Can you work these out from the model? Positions are in its coordinate system, mm. A direction names the side the tool comes from. Coordinates: 2 decimals unless noted, no trailing zeros. Order: outer loops, then holes, each group sorted by start corner. A loop starts at its lowest first (then second) coordinate and runs counter-clockwise, first axis right, second up. Notation, with made-up numbers: (45.25, 75) -> (70.25, 75) arc R16 ccw to (70.25, 87) -> close; hole circle Ø1 at (43.5, 72.5). An arc over 180 degrees is marked (long way). Answer as a JSON object with one key per item and string values. Group by question number.
(1) I want a section at A-A, the plane y = -3.5. List the corners of the cut face in (x, z) for me.
(2) I want a section at D-D, the plane y = 2.75. List the corners of the cut face in (x, z) for me.
(3) I want a section at B-B, the plane x = 19. List the corners of the cut face in (y, z) for me.
(4) If we mould it in two halves opening along Z, with no side actions, what happens to faces 1 (the flat face through (5, -12.83, 8)), 2 (the flat face through (5, -7, 0)), 3 (the cylindrical face through (21.432, -12.826, 7.152)), 4 (the cylindrical face through (5.09, -6.73, 1.27))? For each: pulls with the +Z half, pulls with the -Z half, needs draft (parallel to the pull), parting line crosses it, or undercut.
(5) Which directions (+Z, -Z, +X, -X, +Y, -Y) give clear straight access to the entire face, cutting with the end or side of a thin tool? Please do faces 5 (the flat face through (9.365, 2, 1)), 6 (the flat face through (20.215, -1, 11)), 7 (the flat face through (3, -4, 14.8)), 8 (the flat face through (21, -5, 9.995)), 9 (the flat face through (5, -15.23, 7)).
(6) I want a section at C-C, the plane z = 7.5. List the corners of the cut face in (x, y) for me, plus the area to 3 significant figures.
(7) For pin 1 (1.2 mm diameter, centred on x = 22, y = -5, fed in from -Z); pin 2 (1.6 mm diameter, centred on x = 6, y = -4, fed in from -Z); pin 3 (1.5 mm diameter, centred on x = -8, z = 8.5, fed in from +Y), each with a flat end and sliding along its axis, tell me the tip position at first contact or that it passes through.
(8) I need wall thicknesses on line 1 (X direction, y = 3.5, z = 10.5); line 2 (Z direction, x = -1, y = -9.25); line 3 (Y direction, x = 16.5, z = 11). Which ranges of each line are inside material? Lowest first, please.
from build123d import *

# Parameters (mm, degrees)
F1_DEPTH  = 2.5
F3_DEPTH  = 10.5
F4_W      = 35
F4_H      = 21
F5_DEPTH  = 2
F7_DEPTH  = 2.4
F8_R      = 2
F9_DEPTH  = 25
F10_R     = 2.75
F11_DEPTH = 1.8


with BuildPart() as f1:
    # F0 (on Top) → F1 (new body)
    with BuildSketch(Plane.XY):
        with BuildLine():
            Line((0.864788, 5.76975), (-12.385212, 5.76975))
            Line((-12.385212, 5.76975), (-12.385212, -15.23025))
            Line((-12.385212, -15.23025), (22.614788, -15.23025))
            Line((22.614788, -15.23025), (22.614788, 5.76975))
            Line((22.614788, 5.76975), (9.364788, 5.76975))
            Line((9.364788, 5.76975), (9.364788, -1.989312))
            ThreePointArc((9.364788, -1.989312), (5.114788, -6.239312), (0.864788, -1.989312))
            Line((0.864788, -1.989312), (0.864788, 5.76975))
        make_face()
    extrude(amount=F1_DEPTH)

    # F2 (on face) → F3 (join)
    with BuildSketch(Plane.XY.offset(2.5)):
        Polygon((-9.985212, 5.76975), (-12.385212, 5.76975), (-12.385212, -15.23025), (22.614788, -15.23025), (22.614788, 5.76975), (20.214788, 5.76975), (20.214788, -12.83025), (-9.985212, -12.83025), align=None)
    extrude(amount=F3_DEPTH)

    # F4 (on face) → F5 (join)
    with BuildSketch(Plane.XY.offset(13)):
        with Locations((5.114788, -4.73025)):
            Rectangle(F4_W, F4_H)
    extrude(amount=F5_DEPTH)

    # F6 (on face) → F7 (cut)
    with BuildSketch(Plane.YZ.offset(22.614788)):
        with BuildLine():
            Line((-9.83025, 4), (0.16975, 4))
            ThreePointArc((0.16975, 4), (3.168548, 7.084909), (0, 9.995194))
            Line((0, 9.995194), (-9.660501, 9.995194))
            ThreePointArc((-9.660501, 9.995194), (-12.829049, 7.084909), (-9.83025, 4))
        make_face()
    extrude(amount=-F7_DEPTH, mode=Mode.SUBTRACT)

    # F8 (on face) → F9 (cut)
    with BuildSketch(Plane.XY.offset(15)):
        with Locations((5.114788, -4.73025)):
            Circle(F8_R)
    extrude(amount=-F9_DEPTH, mode=Mode.SUBTRACT)

    # F10 (on face) → F11 (cut)
    with BuildSketch(Plane(origin=(0, 0, 13), x_dir=(1, 0, 0), z_dir=(0, 0, -1))):
        with Locations((5.114788, 4.73025)):
            Circle(F10_R)
    extrude(amount=-F11_DEPTH, mode=Mode.SUBTRACT)


solid = f1.part
Computed values:
{
 "1": {"outline": "(-12.39, 0) -> (1.14, 0) -> (1.14, 2.5) -> (-9.99, 2.5) -> (-9.99, 13) -> (2.66, 13) -> (2.66, 14.8) -> (3.54, 14.8) -> (3.54, 15) -> (-12.39, 15) -> close; (6.69, 14.8) -> (7.57, 14.8) -> (7.57, 13) -> (20.21, 13) -> (20.21, 10) -> (22.61, 10) -> (22.61, 15) -> (6.69, 15) -> close; (9.09, 0) -> (22.61, 0) -> (22.61, 4) -> (20.21, 4) -> (20.21, 2.5) -> (9.09, 2.5) -> close"},
 "2": {"outline": "(-12.39, 0) -> (0.86, 0) -> (0.86, 2.5) -> (-9.99, 2.5) -> (-9.99, 13) -> (20.21, 13) -> (20.21, 8.53) -> (22.61, 8.53) -> (22.61, 15) -> (-12.39, 15) -> close; (9.36, 0) -> (22.61, 0) -> (22.61, 5.47) -> (20.21, 5.47) -> (20.21, 2.5) -> (9.36, 2.5) -> close"},
 "3": {"outline": "(-15.23, 0) -> (5.77, 0) -> (5.77, 2.5) -> (-12.83, 2.5) -> (-12.83, 13) -> (5.77, 13) -> (5.77, 15) -> (-15.23, 15) -> close"},
 "4": {"face 1": "undercut", "face 2": "pulls with the -Z half", "face 3": "undercut", "face 4": "needs draft"},
 "5": {"face 5": "-Z, +Y", "face 6": "+Y", "face 7": "none", "face 8": "+X", "face 9": "+Z, -Z, +X, -X, -Y"},
 "6": {"outline": "(-12.39, -15.23) -> (22.61, -15.23) -> (22.61, -12.79) -> (20.21, -12.79) -> (20.21, -12.83) -> (-9.99, -12.83) -> (-9.99, 5.77) -> (-12.39, 5.77) -> close; (20.21, 3.13) -> (22.61, 3.13) -> (22.61, 5.77) -> (20.21, 5.77) -> close", "area": "135 mm2"},
 "7": {"pin 1": "stops at z = 0", "pin 2": "passes through", "pin 3": "stops at y = -12.83"},
 "8": {"line 1": "x = -12.39 to -9.99, 20.21 to 22.61", "line 2": "z = 0 to 2.5, 13 to 15", "line 3": "y = -15.23 to -12.83"}
}
